```python
from build123d import *

# Parameters (mm, degrees)
ESQUISSE1_R        = 4
ESQUISSE1_R_2      = 0.875
ESQUISSE1_R_3      = 1.5
BOSS_EXTRU_1_DEPTH = 5


with BuildPart() as part:
    # Esquisse1 → Boss.-Extru.1 (new body)
    with BuildSketch(Plane.XY):
        with BuildLine():
            Line((-10.678501768, 2.64), (-4.85386444, 26.2))
            ThreePointArc((-4.85386444, 26.2), (0, 30), (4.85386444, 26.2))
            Line((4.85386444, 26.2), (10.678501768, 2.64))
            ThreePointArc((10.678501768, 2.64), (11, 0), (10.678501768, -2.64))
            Line((10.678501768, -2.64), (4.85386444, -26.2))
            ThreePointArc((4.85386444, -26.2), (0, -30), (-4.85386444, -26.2))
            Line((-4.85386444, -26.2), (-10.678501768, -2.64))
            ThreePointArc((-10.678501768, -2.64), (-11, 0), (-10.678501768, 2.64))
        make_face()
        Circle(ESQUISSE1_R, mode=Mode.SUBTRACT)
        with Locations((7.25, 0)):
            Circle(ESQUISSE1_R_2, mode=Mode.SUBTRACT)
        with Locations((7.25, 3.65)):
            Circle(ESQUISSE1_R_2, mode=Mode.SUBTRACT)
        with Locations(Location((7.25, -3.65, 0), (0, 0, 180))):
            Circle(ESQUISSE1_R_2, mode=Mode.SUBTRACT)
        with Locations((3.65, -7.25)):
            Circle(ESQUISSE1_R_2, mode=Mode.SUBTRACT)
        with Locations((0, -7.25)):
            Circle(ESQUISSE1_R_2, mode=Mode.SUBTRACT)
        with Locations(Location((-3.65, -7.25, 0), (0, 0, 180))):
            Circle(ESQUISSE1_R_2, mode=Mode.SUBTRACT)
        with Locations((-7.25, -3.65)):
            Circle(ESQUISSE1_R_2, mode=Mode.SUBTRACT)
        with Locations((-7.25, 0)):
            Circle(ESQUISSE1_R_2, mode=Mode.SUBTRACT)
        with Locations(Location((-7.25, 3.65, 0), (0, 0, 180))):
            Circle(ESQUISSE1_R_2, mode=Mode.SUBTRACT)
        with Locations((-3.65, 7.25)):
            Circle(ESQUISSE1_R_2, mode=Mode.SUBTRACT)
        with Locations((0, 7.25)):
            Circle(ESQUISSE1_R_2, mode=Mode.SUBTRACT)
        with Locations(Location((3.65, 7.25, 0), (0, 0, 180))):
            Circle(ESQUISSE1_R_2, mode=Mode.SUBTRACT)
        with Locations((0, 25)):
            Circle(ESQUISSE1_R_3, mode=Mode.SUBTRACT)
        with Locations(Location((0, -25, 0), (0, 0, 180))):
            Circle(ESQUISSE1_R_3, mode=Mode.SUBTRACT)
    extrude(amount=BOSS_EXTRU_1_DEPTH)


solid = part.part
```
For this review, take the finished solid that the model builds, in its own axes (mm). Round coordinates to 2 decimals unless told otherwise and drop trailing zeros. Write each loop counter-clockwise with the first axis right and the second up, starting at its lowest first coordinate (ties: lowest second). Pieces come first, ordered by that corner, then holes. Notation, with made-up numbers: M 75.5,25 L 121.5,25 A17 cw 121.5,36 Z; hole C 76,-7 d9. An arc over 180 degrees is marked long. One line per item, written item: value. Start each with the question number.
(1) We need section A-A (y = 0). Give the boundary of the cut face in (x, z) (3 decimals).
(2) We need section C-C (z = 1.55). Count the separate pieces of the cut face and the enclosed holes in it, and give its area (3 significant figures).
(3) The part is to be moulded in two halves that separate along X. For faces 1 (the cylindrical face through (0.195, -26.487, 2.465)), 2 (the cylindrical face through (0, -30, 2)), 3 (the cylindrical face through (11, 0, 2)), 4 (the cylindrical face through (3.76, 6.38, 2.46)), say which applies: released by +X, released by -X, zero draft, split by the parting line, or undercut.
(4) Insertion check: pin 1 (1.6 mm diameter, centred on x = -7.25, y = 3.65, fed in from -Z) (3 decimals); pin 2 (1.5 mm diameter, centred on y = 18, z = 2, fed in from -X); pin 3 (3 mm diameter, centred on y = -6.5, z = 4, fed in from -X); pin 4 (1.5 mm diameter, centred on x = -2.5, z = 1.5, fed in from +Y). Each pin has a flat end and moves straight along its axis. Give the tip position at first contact, or say it passes through.
(5) We need section D-D (y = -25). Give the boundary of the cut face in (x, z), and give its area (3 significant figures).
(6) Wall thickness on line 1 (Y direction, x = 0, z = 2.3) (3 decimals); line 2 (Y direction, x = -0.5, z = 1.35); line 3 (Y direction, x = 3.25, z = 1.25): over which ranges is each line inside the solid? List them lowest first.
(7) We need section B-B (x = 7.25). Give the boundary of the cut face in (y, z) (3 decimals), and give its area (3 significant figures).
Result:
1. outline: M -11,0 L -8.125,0 L -8.125,5 L -11,5 Z; M -6.375,0 L -4,0 L -4,5 L -6.375,5 Z; M 4,0 L 6.375,0 L 6.375,5 L 4,5 Z; M 8.125,0 L 11,0 L 11,5 L 8.125,5 Z
2. separate pieces: 1
2. enclosed holes: 15
2. area: 808 mm²
3. face 1: undercut
3. face 2: split by the parting line
3. face 3: released by +X
3. face 4: undercut
4. pin 1: through
4. pin 2: x = -7.07
4. pin 3: x = -10.1
4. pin 4: y = 29.68
5. outline: M -5.15,0 L -1.5,0 L -1.5,5 L -5.15,5 Z; M 1.5,0 L 5.15,0 L 5.15,5 L 1.5,5 Z
5. area: 36.5 mm²
6. line 1: -30 to -26.5, -23.5 to -8.125, -6.375 to -4, 4 to 6.375, 8.125 to 23.5, 26.5 to 30
6. line 2: -29.97 to -26.41, -23.59 to -7.97, -6.53 to -3.97, 3.97 to 6.53, 7.97 to 23.59, 26.41 to 29.97
6. line 3: -28.8 to -8.03, -6.47 to -2.33, 2.33 to 6.47, 8.03 to 28.8
7. outline: M -16.508,0 L -4.525,0 L -4.525,5 L -16.508,5 Z; M -2.775,0 L -0.875,0 L -0.875,5 L -2.775,5 Z; M 0.875,0 L 2.775,0 L 2.775,5 L 0.875,5 Z; M 4.525,0 L 16.508,0 L 16.508,5 L 4.525,5 Z
7. area: 139 mm²
